```python
from build123d import *

# Parameters (mm, degrees)
BOSS_EXTRUDE1_DEPTH = 121.412
SKETCH2_R           = 2.5796875
CUT_EXTRUDE1_DEPTH  = 12.7


with BuildPart() as part:
    # Sketch1 → Boss-Extrude1 (new body)
    with BuildSketch(Plane.XY):
        Polygon((7.332348419, 0), (3.666174209, 6.35), (-3.666174209, 6.35), (-7.332348419, 0), (-3.666174209, -6.35), (3.666174209, -6.35), align=None)
    extrude(amount=BOSS_EXTRUDE1_DEPTH)

    # Sketch2 → Cut-Extrude1 (cut)
    with BuildSketch(Plane.XY.offset(121.412)):
        Circle(SKETCH2_R)
    cut_extrude1 = extrude(amount=-CUT_EXTRUDE1_DEPTH, mode=Mode.SUBTRACT)

    # Mirror1: Cut-Extrude1 across plane
    add(cut_extrude1.mirror(Plane.XY.offset(60.706)), mode=Mode.SUBTRACT)


solid = part.part
```
The model under review builds one solid part; all positions refer to its coordinate system, in mm. A direction names the side the tool comes from. Round coordinates to 2 decimals unless told otherwise and drop trailing zeros. Write each loop counter-clockwise with the first axis right and the second up, starting at its lowest first coordinate (ties: lowest second). Pieces come first, ordered by that corner, then holes. Notation, with made-up numbers: (71, 8.5) - (121, 8.5) arc R21 ccw to (121, 40.5) - close; hole circle Ø1 at (7, 48). An arc over 180 degrees is marked (long way). Use one line per item in the form item = value.
Q1. Consider section C-C (y = 4). State the section outline as (x, z) points.
Answer key:
outline = (-5.02, 0) - (5.02, 0) - (5.02, 121.41) - (-5.02, 121.41) - close
Q2. Consider section B-B (z = 15.5). State the section outline as (x, y) points.
Answer key:
outline = (-7.33, 0) - (-3.67, -6.35) - (3.67, -6.35) - (7.33, 0) - (3.67, 6.35) - (-3.67, 6.35) - close
Q3. Consider section A-A (x = 0). State the section outline as (y, z) points, and give its area (3 significant figures).
Answer key:
outline = (-6.35, 0) - (-2.58, 0) - (-2.58, 12.7) - (2.58, 12.7) - (2.58, 0) - (6.35, 0) - (6.35, 121.41) - (2.58, 121.41) - (2.58, 108.71) - (-2.58, 108.71) - (-2.58, 121.41) - (-6.35, 121.41) - close
area = 1,410 mm2
Q4. Consider section D-D (x = -5). State the section outline as (y, z) points.
Answer key:
outline = (-4.04, 0) - (4.04, 0) - (4.04, 121.41) - (-4.04, 121.41) - close
Q5. Insertion check: pin 1 Ø3 at (x, y) = (0, 0) entering from -Z; pin 2 Ø2 at (x, y) = (-2.5, -2.5) entering from -Z; pin 3 Ø5 at (y, z) = (-3, 74.5) entering from +X; pin 4 Ø4 at (y, z) = (4, 79.5) entering from +X. Each pin has a flat end and moves straight along its axis. Give the tip position at first contact, or say it passes through.
Answer key:
pin_1 = 12.7
pin_2 = 0
pin_3 = 7.04
pin_4 = 6.18
Q6. Tool access review of faces 1 (the flat face through (0, 0, 12.7)), 2 (the cylindrical face through (-0.56, -2.52, 115.15)), 3 (the flat face through (-5.525, -3.131, 59.856)): name each direction out of +Z, -Z, +X, -X, +Y, -Y from which nothing blocks a thin tool from reaching the whole face with its end or side.
Answer key:
face_1 = -Z
face_2 = +Z
face_3 = +Z, -Z, -X, -Y
Q7. Draft analysis for pull direction X (two halves, no side actions). For faces 4 (the cylindrical face through (-0.56, -2.52, 6.26)), 5 (the flat face through (0, 0, 108.712)), 6 (the flat face through (0, 6.35, 60)), 7 (the flat face through (5.474, -3.219, 59.856)), state which applies: +X half, -X half, draft (parallel to the pull), parting line (faces both ways), or undercut.
Answer key:
face_4 = undercut
face_5 = undercut
face_6 = draft
face_7 = +X half
Q8. For line 1 (Y direction, x = 0, z = 6.5); line 2 (Z direction, x = -2, y = 0.75); line 3 (Y direction, x = -1, z = 112.5), list the stretches that pass through material, from the lowest coordinate up. Write a range as [from, to].
Answer key:
line_1 = [-6.35, -2.58], [2.58, 6.35]
line_2 = [12.7, 108.71]
line_3 = [-6.35, -2.38], [2.38, 6.35]
